Autodesk Inventor part; units mm, degrees
ref_plane "YZ Plane" through (0, 0, 0) normal (1, 0, 0) x (0, 1, 0)
ref_plane "XZ Plane" through (0, 0, 0) normal (0, 1, 0) x (-1, 0, 0)
ref_plane "XY Plane" through (0, 0, 0) normal (0, 0, 1) x (1, 0, 0)
sketch "Sketch1" plane through (0, 0, 0) normal (0, 1, 0) x (-1, 0, 0)
  line L0 (0, 93.9079) -> (150, 93.9079)
  line L1 (150, 93.9079) -> (150, 168.9079)
  line L2 (150, 168.9079) -> (0, 168.9079)
  line L3 (0, 168.9079) -> (0, 93.9079)
  point P0 (0, 0)
  dimension "d0" = 150
  dimension "d1" = 75
extrude "Extrusion1" add sketch "Sketch1" along normal blind 25
sketch "Sketch2" plane through (0, 25, 0) normal (0, 1, 0) x (1, 0, 0)
  line L0 (0, -168.9079) -> (-75, -168.9079)
  line L1 (-75, -156.4079) -> (-112.5, -156.4079)
  line L2 (-75, -156.4079) -> (-37.5, -156.4079)
  line L3 (-37.5, -156.4079) -> (-37.5, -106.4079)
  line L4 (-37.5, -106.4079) -> (-112.5, -106.4079)
  line L5 (-112.5, -106.4079) -> (-112.5, -156.4079)
  point P0 (0, 0)
  dimension "d8" = 37.5
  dimension "d9" = 37.5
  dimension "d10" = 50
  dimension "d11" = 75
extrude "Extrusion2" add sketch "Sketch2" along normal blind 25
sketch "Sketch3" plane through (0, 50, 0) normal (0, 1, 0) x (1, 0, 0)
  line L0 (-112.5, -156.4079) -> (-37.5, -156.4079)
  line L1 (-37.5, -156.4079) -> (-37.5, -131.4079)
  line L2 (-75, -143.4079) -> (-100, -143.4079)
  line L3 (-75, -143.4079) -> (-50, -143.4079)
  line L4 (-50, -143.4079) -> (-50, -119.4079)
  line L5 (-50, -119.4079) -> (-100, -119.4079)
  line L6 (-100, -143.4079) -> (-100, -119.4079)
  point P0 (0, 0)
  dimension "d18" = 25
  dimension "d19" = 25
  dimension "d20" = 24
  dimension "d21" = 50
extrude "Extrusion3" cut sketch "Sketch3" against normal blind 30
sketch "Sketch4" plane through (0, 25, 0) normal (0, 1, 0) x (1, 0, 0)
  line L0 (-37.5, -106.4079) -> (-37.5, -156.4079)
  line L1 (-37.5, -156.4079) -> (-37.5, -131.4079)
  line L2 (-37.5, -131.4079) -> (-37.5, -126.4079)
  line L3 (-37.5, -131.4079) -> (-37.5, -136.4079)
  line L4 (-37.5, -136.4079) -> (0, -136.4079)
  line L5 (0, -168.9079) -> (0, -93.9079)
  line L6 (0, -136.4079) -> (0, -126.4079)
  line L7 (0, -126.4079) -> (-37.5, -126.4079)
  line L8 (-112.5, -156.4079) -> (-112.5, -106.4079)
  line L9 (-112.5, -106.4079) -> (-112.5, -131.4079)
  line L10 (-37.5, -156.4079) -> (-112.5, -156.4079)
  line L11 (-112.5, -131.4079) -> (-112.5, -136.4079)
  line L12 (-112.5, -131.4079) -> (-112.5, -126.4079)
  line L13 (-112.5, -136.4079) -> (-150, -136.4079)
  line L14 (-150, -93.9079) -> (-150, -168.9079)
  line L15 (-150, -136.4079) -> (-150, -126.4079)
  line L16 (-150, -126.4079) -> (-112.5, -126.4079)
  point P0 (0, 0)
  dimension "d25" = 5
  dimension "d26" = 5
  dimension "d27" = 10
  dimension "d29" = 5
  dimension "d30" = 5
  dimension "d31" = 10
extrude "Extrusion4" add sketch "Sketch4" along normal blind 25
sketch "Sketch5" plane through (-150, 25, 136.4079) normal (0, 0, 1) x (1, 0, 0)
  line L0 (37.5, 25) -> (0, 0)
  line L1 (0, 25) -> (37.5, 25)
  line L2 (0, 0) -> (0, 25)
  line L3 (0, 25) -> (37.5, 25)
  point P0 (150, -25)
extrude "Extrusion5" cut sketch "Sketch5" against normal blind 25
sketch "Sketch6" plane through (-37.5, 25, 136.4079) normal (0, 0, 1) x (1, 0, 0)
  line L0 (0, 25) -> (37.5, 25)
  line L1 (37.5, 0) -> (0, 0)
  line L2 (0, 25) -> (37.5, 0)
  line L3 (37.5, 0) -> (37.5, 25)
  line L4 (37.5, 0) -> (37.5, 25)
  line L5 (37.5, 25) -> (0, 25)
  point P0 (37.5, -25)
extrude "Extrusion6" cut sketch "Sketch6" against normal blind 25
sketch "Sketch7" plane through (0, 25, 0) normal (0, 1, 0) x (1, 0, 0)
  line L0 (0, -126.4079) -> (0, -93.9079)
  line L1 (0, -93.9079) -> (-25, -93.9079)
  line L2 (-34, -103.9079) -> (-34, -98.9079)
  line L3 (-34, -103.9079) -> (-34, -108.9079)
  line L4 (-34, -108.9079) -> (-16, -108.9079)
  line L5 (-16, -108.9079) -> (-16, -98.9079)
  line L6 (-16, -98.9079) -> (-34, -98.9079)
  line L7 (-150, -93.9079) -> (-116, -93.9079)
  line L8 (-116, -98.9079) -> (-116, -108.9079)
  line L9 (-116, -108.9079) -> (-134, -108.9079)
  line L10 (-134, -108.9079) -> (-134, -98.9079)
  line L11 (-134, -98.9079) -> (-116, -98.9079)
  line L12 (-116, -153.9079) -> (-116, -163.9079)
  line L13 (-116, -163.9079) -> (-134, -163.9079)
  line L14 (-134, -163.9079) -> (-134, -153.9079)
  line L15 (-134, -153.9079) -> (-116, -153.9079)
  line L16 (-150, -168.9079) -> (0, -168.9079)
  line L17 (-150, -136.4079) -> (-150, -168.9079)
  line L18 (-16, -153.9079) -> (-16, -163.9079)
  line L19 (-16, -163.9079) -> (-34, -163.9079)
  line L20 (-34, -163.9079) -> (-34, -153.9079)
  line L21 (-34, -153.9079) -> (-16, -153.9079)
  line L22 (0, -168.9079) -> (0, -136.4079)
  point P0 (0, 0)
  dimension "d44" = 5
  dimension "d45" = 5
  dimension "d46" = 18
  dimension "d47" = 10
  dimension "d50" = 10
  dimension "d51" = 18
  dimension "d52" = 10
  dimension "d53" = 10
  dimension "d54" = 18
  dimension "d55" = 10
  dimension "d56" = 5
  dimension "d57" = 16
  dimension "d58" = 10
  dimension "d59" = 18
  dimension "d60" = 10
  dimension "d61" = 16
  dimension "d62" = 5
extrude "Extrusion7" cut sketch "Sketch7" against normal blind 25
properties part number "6 - Part 3"
Input: part model. Units: mm. Frame: model coordinates. A direction names the side the tool comes from. Give positions to 0.01 mm unless a question says otherwise; leave off trailing zeros. Loops run counter-clockwise (first coordinate to the right, second up) from the corner with the lowest first, then second, coordinate; pieces in that order, holes last. Notation, with made-up numbers: M -13,9.25 L 22,9.25 A14 ccw 22,29.25 Z; hole C 62.25,38 d4. An arc over 180 degrees is marked long. Use CSV: the item, a comma, the result in double quotes.
(1) Pull-direction query (Y, two-part tool) for faces 6 (the face through (-74, 0, 132)), 7 (the face through (-34, 13, 104)), 8 (the face through (-76, 50, 148)); classes: pulls with the +Y half, pulls with the -Y half, needs draft (parallel to the pull), parting line crosses it, or undercut.
Outcome:
face 6,"pulls with the -Y half"
face 7,"needs draft"
face 8,"pulls with the +Y half"
(2) Material intervals for L1, parallel to X at y = 24, z = 156; L2, parallel to Z at x = -67, y = 41.5; L3, parallel to Z at x = -60, y = 20.5, sorted ascending. Write a range as [from, to].
Outcome:
L1,"x = [-150, -134], [-116, -34], [-16, 0]"
L2,"z = [106.41, 119.41], [143.41, 156.41]"
L3,"z = [93.91, 119.41], [143.41, 168.91]"
(3) Section A-A, the plane y = 14.5. Return loops of the section in (x, z).
Outcome:
outline,"M -150,93.91 L 0,93.91 L 0,168.91 L -150,168.91 Z; hole M -134,98.91 L -116,98.91 L -116,108.91 L -134,108.91 Z; hole M -134,153.91 L -116,153.91 L -116,163.91 L -134,163.91 Z; hole M -34,98.91 L -16,98.91 L -16,108.91 L -34,108.91 Z; hole M -34,153.91 L -16,153.91 L -16,163.91 L -34,163.91 Z"
(4) Section D-D, the plane x = -105. Return loops of the section in (y, z), plus the area to 4 significant figures.
Outcome:
outline,"M 0,93.91 L 25,93.91 L 25,106.41 L 50,106.41 L 50,156.41 L 25,156.41 L 25,168.91 L 0,168.91 Z"
area,"3,125 mm²"
(5) Pin query (flat end, axial travel): P1, Ø10, axis at y = 36.5, z = 115.5, coming from the +X side; P2, Ø2, axis at x = -54.5, y = 29, coming from the -Z side; P3, Ø16, axis at y = 38, z = 149, coming from the -X side. Return the tip coordinate at first contact, or that it passes through.
Outcome:
P1,"stops at x = -37.5"
P2,"stops at z = 106.41"
P3,"stops at x = -112.5"
(6) Section C-C, the plane z = 158.5. Return loops of the section in (x, y), plus the area to 3 significant figures.
Outcome:
outline,"M -150,0 L -134,0 L -134,25 L -150,25 Z; M -116,0 L -34,0 L -34,25 L -116,25 Z; M -16,0 L 0,0 L 0,25 L -16,25 Z"
area,"2,850 mm²"
(7) Section B-B, the plane y = 21.5. Return loops of the section in (x, z), plus the area to 3 significant figures.
Outcome:
outline,"M -150,93.91 L 0,93.91 L 0,168.91 L -150,168.91 Z; hole M -134,98.91 L -116,98.91 L -116,108.91 L -134,108.91 Z; hole M -134,153.91 L -116,153.91 L -116,163.91 L -134,163.91 Z; hole M -100,119.41 L -50,119.41 L -50,143.41 L -100,143.41 Z; hole M -34,98.91 L -16,98.91 L -16,108.91 L -34,108.91 Z; hole M -34,153.91 L -16,153.91 L -16,163.91 L -34,163.91 Z"
area,"9,330 mm²"
(8) Set-up query: faces 1 (the face through (-27, 32, 126.408)), 2 (the face through (-76, 37, 156.408)), 3 (the face through (-112.5, 37, 116)), 4 (the face through (-112.5, 37, 146)), 5 (the face through (-25, 13, 98.908)). Return all of +Z, -Z, +X, -X, +Y, -Y with unobstructed straight access to the full face (end or side cutting, diameter ignored); none if empty.
Outcome:
face 1,"-Z, +X, +Y"
face 2,"+Z, +X, -X, +Y"
face 3,"-Z, -X, +Y"
face 4,"+Z, -X, +Y"
face 5,"+Y, -Y"
